```python
from build123d import *

# Parameters (mm, degrees)
SKETCH_1_W          = 40
SKETCH_1_H          = 60
EXTRUDE_1_DEPTH     = 350
CHAMFER_1_SIZE      = 10
HOLE_WIZARD_M16_1_D = 14
CHAMFER_2_SIZE      = 5


with BuildPart() as part:
    # 草图1 → 凸台-拉伸1 (new body)
    with BuildSketch(Plane.XY):
        with Locations((20, -30)):
            Rectangle(SKETCH_1_W, SKETCH_1_H)
    extrude(amount=EXTRUDE_1_DEPTH)

    # 倒角1
    chamfer_1_edges = [part.edges().sort_by_distance(p)[0] for p in [
        (40, 0, 175),
        (0, -60, 175),
    ]]
    chamfer(chamfer_1_edges, length=CHAMFER_1_SIZE)

    # M16 螺纹孔1 (through all)
    with Locations(Plane(origin=(0, 0, 0), x_dir=(1, 0, 0), z_dir=(0, 1, 0))):
        with Locations((20, -315), (20, -175), (20, -35)):
            Hole(HOLE_WIZARD_M16_1_D / 2)

    # 倒角2
    chamfer_2_edges = [part.edges().sort_by_distance(p)[0] for p in [
        (40, -35, 350),
        (0, -25, 350),
        (40, -35, 0),
        (0, -25, 0),
    ]]
    chamfer(chamfer_2_edges, length=CHAMFER_2_SIZE)


solid = part.part
```
Geometry check sheet. Reference: the model listing, model coordinates, mm. Coordinates: 2 decimals unless noted, no trailing zeros. Write each loop counter-clockwise with the first axis right and the second up, starting at its lowest first coordinate (ties: lowest second). Pieces come first, ordered by that corner, then holes. Notation, with made-up numbers: (-2, -20.5) -> (10, -20.5) arc R27 cw to (10, 10.5) -> close; hole circle Ø9 at (-21.5, 26). An arc over 180 degrees is marked (long way). Use CSV: the item, a comma, the result in double quotes. Start each with the question number.
Item 1: Thickness scan on line 1 (Z direction, x = 20, y = -33); line 2 (X direction, y = -33, z = 315); line 3 (X direction, y = -53.5, z = 230). Record the ranges inside material, lowest first.
Item 2: Cross-section at A-A, the plane y = -45.5. Record the cut outline in (x, z).
Item 3: Cross-section at C-C, the plane x = 20. Record the cut outline in (y, z).
Item 4: Mould release check, pull along X, two halves, no side actions. Record for faces 1 (the flat face through (20, -30, 350)), 2 (the cylindrical face through (20.91, -30.42, 28.06)), 3 (the flat face through (0, -25, 173)): released by +X, released by -X, zero draft, split by the parting line, or undercut.
Item 5: Cross-section at B-B, the plane z = 175. Record the cut outline in (x, y).
Answers:
1,line 1,"0 to 28, 42 to 168, 182 to 308, 322 to 350"
1,line 2,"0 to 13, 27 to 40"
1,line 3,"3.5 to 40"
2,outline,"(0, 5) -> (5, 0) -> (35, 0) -> (40, 5) -> (40, 345) -> (35, 350) -> (5, 350) -> (0, 345) -> close; hole circle Ø14 at (20, 35); hole circle Ø14 at (20, 175); hole circle Ø14 at (20, 315)"
3,outline,"(-60, 0) -> (0, 0) -> (0, 28) -> (-60, 28) -> close; (-60, 42) -> (0, 42) -> (0, 168) -> (-60, 168) -> close; (-60, 182) -> (0, 182) -> (0, 308) -> (-60, 308) -> close; (-60, 322) -> (0, 322) -> (0, 350) -> (-60, 350) -> close"
4,face 1,"zero draft"
4,face 2,"undercut"
4,face 3,"released by -X"
5,outline,"(0, -50) -> (10, -60) -> (13, -60) -> (13, 0) -> (0, 0) -> close; (27, -60) -> (40, -60) -> (40, -10) -> (30, 0) -> (27, 0) -> close"
